Work out the finished part from the listing and answer in its coordinate system (mm). A direction names the side the tool comes from. Give positions to 0.01 mm unless a question says otherwise; leave off trailing zeros. Loops run counter-clockwise (first coordinate to the right, second up) from the corner with the lowest first, then second, coordinate; pieces in that order, holes last. Notation, with made-up numbers: (23.25, 89.25) - (39.25, 89.25) arc R21 ccw to (39.25, 98.25) - close; hole circle Ø9 at (25, 87.25). An arc over 180 degrees is marked (long way). One line per item, written item: value.
Autodesk Inventor part; units mm, degrees
ref_plane "YZ Plane" through (0, 0, 0) normal (1, 0, 0) x (0, 1, 0)
ref_plane "XZ Plane" through (0, 0, 0) normal (0, 1, 0) x (-1, 0, 0)
ref_plane "XY Plane" through (0, 0, 0) normal (0, 0, 1) x (1, 0, 0)
sketch "Sketch1" plane through (0, 0, 0) normal (0, 1, 0) x (-1, 0, 0)
  line L0 (24.2857, 221.4286) -> (-135.7143, 221.4286)
  line L1 (-135.7143, 221.4286) -> (-135.7143, -28.5714)
  line L2 (-135.7143, -28.5714) -> (24.2857, -28.5714)
  line L3 (24.2857, -28.5714) -> (24.2857, 221.4286)
  circle A0 centre (-55.7143, -38.5714) radius 80
  line L4 (24.2857, -28.5714) -> (24.2857, -38.5714)
  line L5 (-135.7143, -28.5714) -> (-135.7143, -38.5714)
  point P0 (0, 0)
  dimension "d0" = 250
  dimension "d1" = 160
  dimension "d2" = 160
  dimension "d8" = 10
extrude "Extrusion1" add sketch "Sketch1" along normal blind 30
sketch "Sketch2" plane through (0, 30, 0) normal (0, 1, 0) x (1, 0, 0)
  arc A0 (135.7143, 38.5714) -> (-24.2857, 38.5714) centre (55.7143, 38.5714) ccw
  circle A1 centre (55.7143, 38.5714) radius 75
  point P0 (0, 0)
  dimension "d5" = 150
extrude "Extrusion2" cut sketch "Sketch2" against normal blind 40
sketch "Sketch3" plane through (0, 30, 0) normal (0, 1, 0) x (1, 0, 0)
  circle A0 centre (55.7143, 38.5714) radius 75
  circle A1 centre (55.7143, 38.5714) radius 75
  line L0 (152, 38.5714) -> (103.8571, -44.8144)
  line L1 (103.8571, -44.8144) -> (7.5714, -44.8144)
  line L2 (7.5714, -44.8144) -> (-40.5714, 38.5714)
  line L3 (-40.5714, 38.5714) -> (7.5714, 121.9573)
  line L4 (7.5714, 121.9573) -> (103.8571, 121.9573)
  line L5 (103.8571, 121.9573) -> (152, 38.5714)
  line L6 (140, 38.5714) -> (97.8571, -34.4221)
  line L7 (97.8571, -34.4221) -> (13.5714, -34.4221)
  line L8 (13.5714, -34.4221) -> (-28.5714, 38.5714)
  line L9 (-28.5714, 38.5714) -> (13.5714, 111.565)
  line L10 (13.5714, 111.565) -> (97.8571, 111.565)
  line L11 (97.8571, 111.565) -> (140, 38.5714)
  circle A2 centre (140, 38.5714) radius 5
  circle A3 centre (97.8571, 111.565) radius 5
  circle A4 centre (13.5714, 111.565) radius 5
  circle A5 centre (-28.5714, 38.5714) radius 5
  circle A6 centre (13.5714, -34.4221) radius 5
  circle A7 centre (97.8571, -34.4221) radius 5
  point P0 (0, 0)
  dimension "d15" = 360
sketch "Sketch4" plane through (0, 0, 0) normal (0, -1, 0) x (1, 0, 0)
  circle A0 centre (55.7143, -38.5714) radius 75
  circle A1 centre (55.7143, -38.5714) radius 75
  circle A2 centre (55.7143, -38.5714) radius 47
  dimension "d9" = 94
  dimension "d10" = 150
extrude "Extrusion3" add sketch "Sketch4" against normal blind 5
sketch "Sketch5" plane through (0, 30, 0) normal (0, 1, 0) x (1, 0, 0)
  circle A0 centre (55.7143, 38.5714) radius 75
  circle A1 centre (55.7143, 38.5714) radius 75
  line L0 (152, 38.5714) -> (103.8571, -44.8144)
  line L1 (103.8571, -44.8144) -> (7.5714, -44.8144)
  line L2 (7.5714, -44.8144) -> (-40.5714, 38.5714)
  line L3 (-40.5714, 38.5714) -> (7.5714, 121.9573)
  line L4 (7.5714, 121.9573) -> (103.8571, 121.9573)
  line L5 (103.8571, 121.9573) -> (152, 38.5714)
  line L6 (140, 38.5714) -> (97.8571, -34.4221)
  line L7 (97.8571, -34.4221) -> (13.5714, -34.4221)
  line L8 (13.5714, -34.4221) -> (-28.5714, 38.5714)
  line L9 (-28.5714, 38.5714) -> (13.5714, 111.565)
  line L10 (13.5714, 111.565) -> (97.8571, 111.565)
  line L11 (97.8571, 111.565) -> (140, 38.5714)
  circle A2 centre (140, 38.5714) radius 5
  circle A3 centre (97.8571, 111.565) radius 5
  circle A4 centre (13.5714, 111.565) radius 5
  circle A5 centre (-28.5714, 38.5714) radius 5
  circle A6 centre (13.5714, -34.4221) radius 5
  circle A7 centre (97.8571, -34.4221) radius 5
  arc A8 (135.7143, 38.5714) -> (-24.2857, 38.5714) centre (55.7143, 38.5714) ccw
  circle A9 centre (55.7143, 38.5714) radius 2.2469
  point P0 (0, 0)
  point P1 (0, 0)
  dimension "d19" = 360
extrude "Extrusion4" cut sketch "Sketch5" against normal blind 30 contours A2 L11 L6 | L6 L11 A2 | A7 L7 L6 | L6 L7 A7 | A3 A8 L10 L11 | L11 L10 A3 | A3 A8 | A6 L8 L7 | L7 L8 A6 | A4 A8 L9 L10 | L10 L9 A4 | A4 A8 | A5 L9 L8 | L8 L9 A5
extrude "Extrusion5" add sketch "Sketch3" against normal blind 30 contours A0 L11 A2 L6 | A0 L10 A3 L11 | L6 A7 L7 A0 | A0 L9 A4 L10 | L7 A6 L8 A0 | A0 L8 A5 L9 | L0 L1 L2 L3 L4 L5
fillet "Fillet1" radius 12 6 edges at (103.8571, 15, -121.9573) (152, 15, -38.5714) (7.5714, 15, -121.9573) (-40.5714, 15, -38.5714) (-24.2857, 15, -10.3637) (135.7143, 15, -10.3637)
sketch "Sketch6" plane through (0, 30, 0) normal (0, 1, 0) x (1, 0, 0)
  circle A0 centre (13.5714, 111.565) radius 5
  circle A1 centre (97.8571, 111.565) radius 5
  circle A2 centre (-28.5714, 38.5714) radius 5
  circle A3 centre (140, 38.5714) radius 5
  circle A4 centre (55.7143, 38.5714) radius 75
  circle A5 centre (97.8571, -34.4221) radius 5
  circle A6 centre (13.5714, -34.4221) radius 5
  arc A7 (-37.1073, 44.5714) -> (-37.1073, 32.5714) centre (-26.715, 38.5714) ccw
  line L0 (-37.1073, 32.5714) -> (-25.8934, 13.1484)
  arc A8 (-24.2857, 7.1484) -> (-25.8934, 13.1484) centre (-36.2857, 7.1484) ccw
  line L1 (-24.2857, 7.1484) -> (-24.2857, -221.4286)
  line L2 (-24.2857, -221.4286) -> (135.7143, -221.4286)
  line L3 (135.7143, -221.4286) -> (135.7143, 7.1484)
  arc A9 (137.322, 13.1484) -> (135.7143, 7.1484) centre (147.7143, 7.1484) ccw
  line L4 (137.322, 13.1484) -> (148.5359, 32.5714)
  arc A10 (148.5359, 32.5714) -> (148.5359, 44.5714) centre (138.1436, 38.5714) ccw
  line L5 (148.5359, 44.5714) -> (107.3212, 115.9573)
  arc A11 (107.3212, 115.9573) -> (96.9289, 121.9573) centre (96.9289, 109.9573) ccw
  line L6 (96.9289, 121.9573) -> (14.4996, 121.9573)
  arc A12 (14.4996, 121.9573) -> (4.1073, 115.9573) centre (14.4996, 109.9573) ccw
  line L7 (4.1073, 115.9573) -> (-37.1073, 44.5714)
  line L8 (-4.2857, -201.4286) -> (-4.2857, 7.1484)
  arc A13 (-4.2857, 7.1484) -> (-8.5729, 23.1484) centre (-36.2857, 7.1484) ccw
  line L9 (-8.5729, 23.1484) -> (-17.4774, 38.5714)
  line L10 (-17.4774, 38.5714) -> (19.1184, 101.9573)
  line L11 (19.1184, 101.9573) -> (92.3101, 101.9573)
  line L12 (92.3101, 101.9573) -> (128.906, 38.5714)
  line L13 (128.906, 38.5714) -> (120.0015, 23.1484)
  arc A14 (120.0015, 23.1484) -> (115.7143, 7.1484) centre (147.7143, 7.1484) ccw
  line L14 (115.7143, 7.1484) -> (115.7143, -201.4286)
  line L15 (115.7143, -201.4286) -> (-4.2857, -201.4286)
  circle A15 centre (55.7143, 38.5714) radius 95
  point P0 (0, 0)
  point P1 (115.7143, -35.0832)
  point P2 (-4.2857, -35.0832)
  dimension "d25" = 20
  dimension "d26" = 190
extrude "Extrusion6" cut sketch "Sketch6" against normal blind 5 contours A15 L14 L15 L8
sketch "Sketch7" plane through (0, 30, 0) normal (0, 1, 0) x (1, 0, 0)
  circle A0 centre (55.7143, 38.5714) radius 75
  circle A1 centre (55.7143, 38.5714) radius 79.2857
  circle A2 centre (-28.5714, 38.5714) radius 5
  circle A3 centre (55.7143, 38.5714) radius 75
  point P0 (0, 0)
  dimension "d29" = 150
extrude "Extrusion7" add sketch "Sketch7" along normal blind 10 contours A1
sketch "Sketch8" plane through (0, 30, 0) normal (0, 1, 0) x (1, 0, 0)
  circle A0 centre (55.7143, -45.7146) radius 5
  circle A1 centre (55.7143, 38.5714) radius 47
  circle A2 centre (77.5291, -42.8426) radius 5
  circle A3 centre (97.8573, -34.4224) radius 5
  circle A4 centre (115.3135, -21.0278) radius 5
  circle A5 centre (128.7081, -3.5716) radius 5
  circle A6 centre (137.1283, 16.7566) radius 5
  circle A7 centre (140.0003, 38.5714) radius 5
  circle A8 centre (137.1283, 60.3863) radius 5
  circle A9 centre (128.7081, 80.7144) radius 5
  circle A10 centre (115.3135, 98.1706) radius 5
  circle A11 centre (97.8573, 111.5652) radius 5
  circle A12 centre (77.5291, 119.9855) radius 5
  circle A13 centre (55.7143, 122.8574) radius 5
  circle A14 centre (33.8995, 119.9855) radius 5
  circle A15 centre (13.5713, 111.5652) radius 5
  circle A16 centre (-3.8849, 98.1706) radius 5
  circle A17 centre (-17.2795, 80.7144) radius 5
  circle A18 centre (-25.6997, 60.3863) radius 5
  circle A19 centre (-28.5717, 38.5714) radius 5
  circle A20 centre (-25.6997, 16.7566) radius 5
  circle A21 centre (-17.2795, -3.5716) radius 5
  circle A22 centre (-3.8849, -21.0278) radius 5
  circle A23 centre (13.5713, -34.4224) radius 5
  circle A24 centre (33.8995, -42.8426) radius 5
  point P0 (0, 0)
  dimension "d32" = 84.286
  dimension "d35" = 360
  dimension "d39" = 10
extrude "Extrusion8" cut sketch "Sketch8" against normal blind 35 contours A0 | A2 | A4 | A5 | A21 | A22 | A24
sketch "Sketch9" plane through (0, 25, 0) normal (0, 1, 0) x (1, 0, 0)
  line L0 (135.7143, -221.4286) -> (135.7143, 7.1484)
  line L1 (-24.2857, -221.4286) -> (135.7143, -221.4286)
  line L2 (-24.2857, 7.1484) -> (-24.2857, -221.4286)
  circle A0 centre (55.7143, -141.4286) radius 80
  circle A1 centre (55.7143, -141.4286) radius 42.5
  point P0 (0, 0)
  dimension "d40" = 85
extrude "Extrusion9" cut sketch "Sketch9" against normal blind 40 contours A1
sketch "Sketch10" plane through (0, 0, 0) normal (0, -1, 0) x (1, 0, 0)
  circle A0 centre (-17.2795, 3.5716) radius 5
  circle A1 centre (128.7081, 3.5716) radius 5
  point P0 (0, 0)
extrude "Extrusion10" add sketch "Sketch10" against normal blind 30
properties part number "PatronDerzavka" material "Aluminum 6061"
1. Flat-ended cylindrical pins translate along their axes: pin 1 Ø4 at (y, z) = (27.5, 145.5) entering from +X; pin 2 Ø1 at (y, z) = (30, -84) entering from +X; pin 3 Ø4 at (y, z) = (29, 49.5) entering from -X. Find the tip coordinate at first contact, or state that the pin passes through.
Output:
pin 1: stops at x = 135.71
pin 2: stops at x = 126.06
pin 3: stops at x = -24.29
2. For faces 5 (the cylindrical face through (52.029, 15.21, 42.335)), 6 (the flat face through (-24.286, 15, 106)), determine the directions among +Z, -Z, +X, -X, +Y, -Y from which every point of the face is accessible in a straight line to the end or side of a thin tool.
Output:
face 5: +Y, -Y
face 6: +Z, -X, +Y, -Y
3. The mould has two halves that part along X. Classify faces 1 (the cylindrical face through (136.11, 14.79, -10.21)), 2 (the flat face through (54.9, 25, 98.6)), 3 (the cylindrical face through (-24.683, 15.21, -10.212)), 4 (the flat face through (55, 15, 221.429)): released by +X, released by -X, zero draft, split by the parting line, or undercut.
Output:
face 1: released by +X
face 2: undercut
face 3: released by -X
face 4: zero draft
4. Section C-C (y = 17) is taken. Count the separate pieces of the cut face and the enclosed holes in it, and give its area (3 significant figures).
Output:
separate pieces: 1
enclosed holes: 13
area: 29,900 mm²
5. Find the intervals of material crossed by line 1 along Z through (x, y) = (55, 17.5); line 2 along Z through (x, y) = (72, 13.5); line 3 along Z through (x, y) = (87.5, 8.5), in increasing order.
Output:
line 1: z = -121.96 to -113.57, 36.43 to 40.77, 50.66 to 98.93, 183.92 to 221.43
line 2: z = -121.96 to -111.78, 34.64 to 102.17, 180.68 to 221.43
line 3: z = -121.96 to -106.5, 29.36 to 113.22, 169.64 to 221.43
6. Section A-A (x = 22) is taken. Write down the section's boundary in (y, z), and give its area (3 significant figures).
Output:
outline: (0, -121.96) - (30, -121.96) - (30, -110.33) - (40, -110.33) - (40, -105.57) - (5, -105.57) - (5, -71.32) - (0, -71.32) - close; (0, -5.82) - (5, -5.82) - (5, 28.42) - (40, 28.42) - (40, 33.19) - (30, 33.19) - (30, 50.24) - (25, 50.24) - (25, 115.55) - (0, 115.55) - close; (0, 167.31) - (25, 167.31) - (25, 201.43) - (30, 201.43) - (30, 221.43) - (0, 221.43) - close
area: 4,670 mm²
7. Section D-D (z = 65) is taken. Write down the section's boundary in (x, y), and give its area (3 significant figures).
Output:
outline: (-24.29, 0) - (135.71, 0) - (135.71, 30) - (115.71, 30) - (115.71, 25) - (-4.29, 25) - (-4.29, 30) - (-24.29, 30) - close
area: 4,200 mm²
8. Section B-B (z = 133) is taken. Write down the section's boundary in (x, y).
Output:
outline: (-24.29, 0) - (14.06, 0) - (14.06, 25) - (-4.29, 25) - (-4.29, 30) - (-24.29, 30) - close; (97.37, 0) - (135.71, 0) - (135.71, 30) - (115.71, 30) - (115.71, 25) - (97.37, 25) - close
